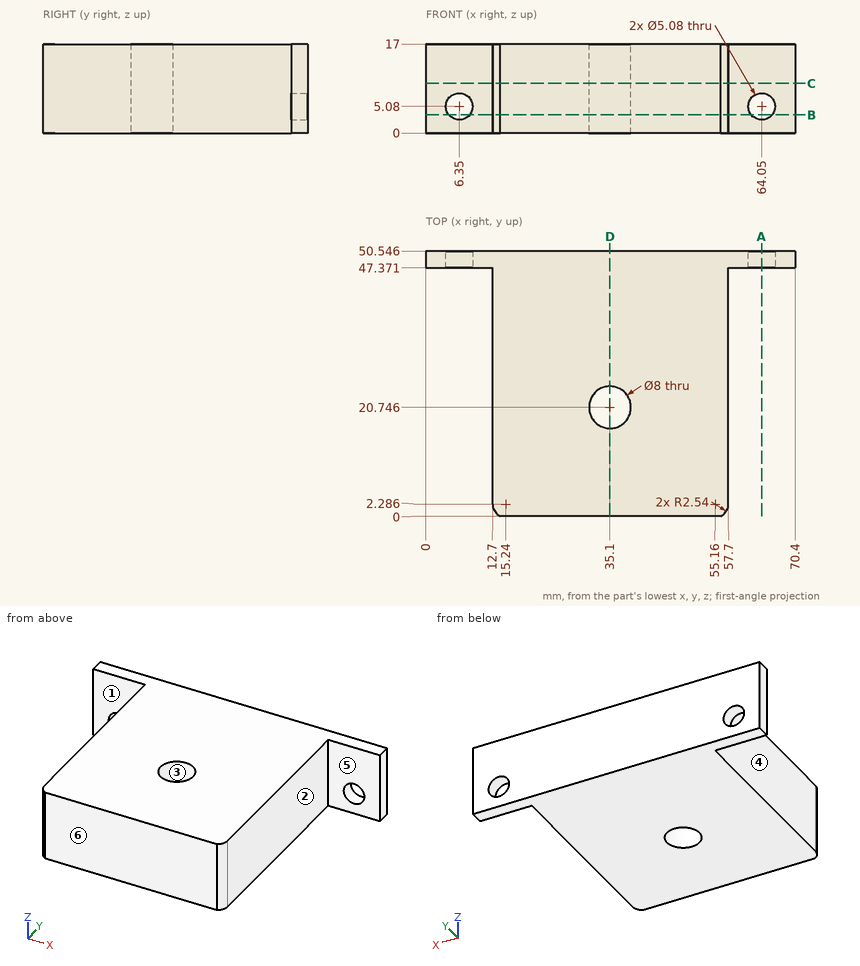
Job drawing, mm, ordinate dimensions from the low corner. One solid piece. A direction names the side the tool comes from. Give positions to 0.01 mm unless a question says otherwise; leave off trailing zeros. Order: outer loops, then holes, each group sorted by start corner. A loop starts at its lowest first (then second) coordinate and runs counter-clockwise, first axis right, second up. Notation, with made-up numbers: (59.5, 61) - (77.5, 61) arc R29 ccw to (77.5, 91) - close; hole circle Ø1 at (83.25, -10.75). An arc over 180 degrees is marked (long way). Answer in a Markdown table with one row per item.
1. Saw through at A-A, the plane x = 64.05. Give the cut face in (y, z), plus the area to 3 significant figures.
Data:
| item | result |
|---|---|
| outline | (47.37, 0) - (50.55, 0) - (50.55, 2.54) - (47.37, 2.54) - close; (47.37, 7.62) - (50.55, 7.62) - (50.55, 17) - (47.37, 17) - close |
| area | 37.8 mm² |
2. Saw through at C-C, the plane z = 9.5. Give the cut face in (x, y), plus the area to 3 significant figures.
Data:
| item | result |
|---|---|
| outline | (0, 47.37) - (12.7, 47.37) - (12.7, 2.29) arc R2.54 ccw to (14.13, 0) - (56.27, 0) arc R2.54 ccw to (57.7, 2.29) - (57.7, 47.37) - (70.4, 47.37) - (70.4, 50.55) - (0, 50.55) - close; hole circle Ø8 at (35.1, 20.75) |
| area | 2,300 mm² |
3. Saw through at B-B, the plane z = 3.5. Give the cut face in (x, y).
Data:
| item | result |
|---|---|
| outline | (0, 47.37) - (4.36, 47.37) - (4.36, 50.55) - (0, 50.55) - close; (8.34, 47.37) - (12.7, 47.37) - (12.7, 2.29) arc R2.54 ccw to (14.13, 0) - (56.27, 0) arc R2.54 ccw to (57.7, 2.29) - (57.7, 47.37) - (62.06, 47.37) - (62.06, 50.55) - (8.34, 50.55) - close; (66.04, 47.37) - (70.4, 47.37) - (70.4, 50.55) - (66.04, 50.55) - close; hole circle Ø8 at (35.1, 20.75) |
4. Flat gauge pins, fed straight in: pin 1 (5 mm diameter, centred on y = 29.5, z = 11.5, fed in from -X); pin 2 (1.5 mm diameter, centred on y = 21, z = 14, fed in from +X); pin 3 (10 mm diameter, centred on x = 64, z = 8, fed in from -Y). Where does each tip first touch, or does it go through?
Data:
| item | result |
|---|---|
| pin 1 | stops at x = 12.7 |
| pin 2 | stops at x = 57.7 |
| pin 3 | stops at y = 47.37 |
5. Pull direction Y, two halves, no side cores. Call the marked faces 1, 2 and 3: pulls with the +Y half, pulls with the -Y half, needs draft (parallel to the pull), parting line crosses it, or undercut.
Data:
| item | result |
|---|---|
| face 1 | pulls with the -Y half |
| face 2 | needs draft |
| face 3 | undercut |
6. Tool access for the marked faces 4, 5 and 6: list every direction of +Z, -Z, +X, -X, +Y, -Y with a clear straight run to the whole face (end or side of a thin tool).
Data:
| item | result |
|---|---|
| face 4 | +Z, -Z, -X, -Y |
| face 5 | +Z, -Z, +X, -Y |
| face 6 | +Z, -Z, +X, -X, -Y |
7. Probe probe 1 along X at (y, z) = (49.65, 5.08); probe 2 along Z at (x, y) = (64.05, 48.6); probe 3 along Y at (x, z) = (35.1, 8.5). List the from-to ranges inside material, lowest first. Write a range as [from, to].
Data:
| item | result |
|---|---|
| probe 1 | x = [0, 3.81], [8.89, 61.51], [66.59, 70.4] |
| probe 2 | z = [0, 2.54], [7.62, 17] |
| probe 3 | y = [0, 16.75], [24.75, 50.55] |
8. Saw through at D-D, the plane x = 35.1. Give the cut face in (y, z), plus the area to 3 significant figures.
Data:
| item | result |
|---|---|
| outline | (0, 0) - (16.75, 0) - (16.75, 17) - (0, 17) - close; (24.75, 0) - (50.55, 0) - (50.55, 17) - (24.75, 17) - close |
| area | 723 mm² |
